```python
from build123d import *

# Parameters (mm, degrees)
BOSS_EXTRUDE1_DEPTH = 0.8
SKETCH3_R           = 0.5
CUT_EXTRUDE1_DEPTH  = 1.8


with BuildPart() as part:
    # Sketch2 → Boss-Extrude1 (new body)
    with BuildSketch(Plane.XY):
        with BuildLine():
            Line((-4.074883717, 6.236811902), (-2.980955202, 4.562499982))
            ThreePointArc((-2.980955202, 4.562499982), (0, -5.45), (2.980955202, 4.562499982))
            Line((2.980955202, 4.562499982), (4.074883717, 6.236811902))
            Line((4.074883717, 6.236811902), (2.400571797, 7.330740416))
            Line((2.400571797, 7.330740416), (0.5, 4.421820892))
            ThreePointArc((0.5, 4.421820892), (0, -4.45), (-0.5, 4.421820892))
            Line((-0.5, 4.421820892), (-2.400571797, 7.330740416))
            Line((-2.400571797, 7.330740416), (-4.074883717, 6.236811902))
        make_face()
    extrude(amount=BOSS_EXTRUDE1_DEPTH)

    # Sketch3 → Cut-Extrude1 (cut, through all)
    with BuildSketch(Plane.XY.offset(0.8)):
        with Locations((-2.6907635, 5.946620199)):
            Circle(SKETCH3_R)
        with Locations((2.6907635, 5.946620199)):
            Circle(SKETCH3_R)
    extrude(amount=-CUT_EXTRUDE1_DEPTH, mode=Mode.SUBTRACT)


solid = part.part
```
Verification items for the finished model (mm, model axes). A direction names the side the tool comes from. Give positions to 0.01 mm unless a question says otherwise; leave off trailing zeros. Loops run counter-clockwise (first coordinate to the right, second up) from the corner with the lowest first, then second, coordinate; pieces in that order, holes last.
1. Section check C-C, the plane x = 0. Enter the section's corners in (y, z), then the cut area to 3 significant figures.
2. Mould release check, pull along Y, two halves, no side actions. Record for faces 6 (the cylindrical face through (0.189, -4.446, 0.394)), 7 (the flat face through (-3.23, 6.79, 0.39)), 8 (the flat face through (-1.2, 4.8, 0.8)): released by +Y, released by -Y, zero draft, split by the parting line, or undercut.
3. Section check B-B, the plane z = 0.15. Enter the section's corners in (x, y), then the cut area to 3 significant figures.
4. Set-up check for faces 1 (the cylindrical face through (-0.196, -5.446, 0.394)), 2 (the flat face through (3.52, 5.39, 0.39)), 3 (the flat face through (-3.536, 5.411, 0.394)), 4 (the flat face through (-1.2, 4.8, 0)), 5 (the flat face through (-1.44, 5.86, 0.39)): record each of +Z, -Z, +X, -X, +Y, -Y from which the full face is reachable in a straight line by a thin tool's end or side.
5. Section check A-A, the plane y = 0. Enter the section's corners in (x, z), then the cut area to 3 significant figures.
6. Thickness scan on line 1 (X direction, y = 0, z = 0.6); line 2 (Y direction, x = 3.75, z = 0.55); line 3 (Y direction, x = 2.25, z = 0.1). Record the ranges inside material, lowest first.
7. Section check D-D, the plane y = 4.25. Enter the section's corners in (x, z), then the cut area to 3 significant figures.
Geometry says:
1. outline: (-5.45, 0) - (-4.45, 0) - (-4.45, 0.8) - (-5.45, 0.8) - close
1. area: 0.800 mm2
2. face 6: undercut
2. face 7: released by +Y
2. face 8: zero draft
3. outline: (-4.07, 6.24) - (-2.98, 4.56) arc R5.45 ccw (long way) to (2.98, 4.56) - (4.07, 6.24) - (2.4, 7.33) - (0.5, 4.42) arc R4.45 cw (long way) to (-0.5, 4.42) - (-2.4, 7.33) - close; hole circle Ø1 at (-2.69, 5.95); hole circle Ø1 at (2.69, 5.95)
3. area: 36.4 mm2
4. face 1: +Z, -Z
4. face 2: +Z, -Z, +X
4. face 3: +Z, -Z, -X
4. face 4: -Z, +X, -X, +Y, -Y
4. face 5: +Z, -Z, +Y
5. outline: (-5.45, 0) - (-4.45, 0) - (-4.45, 0.8) - (-5.45, 0.8) - close; (4.45, 0) - (5.45, 0) - (5.45, 0.8) - (4.45, 0.8) - close
5. area: 1.60 mm2
6. line 1: x = -5.45 to -4.45, 4.45 to 5.45
6. line 2: y = -3.95 to -2.4, 2.4 to 3.95, 5.74 to 6.45
6. line 3: y = -4.96 to -3.84, 3.84 to 5.71, 6.18 to 7.1
7. outline: (-3.41, 0) - (-1.32, 0) - (-1.32, 0.8) - (-3.41, 0.8) - close; (1.32, 0) - (3.41, 0) - (3.41, 0.8) - (1.32, 0.8) - close
7. area: 3.35 mm2
